Check sheet for the modelled part. Datum: model origin and axes. Units: mm. Face numbers are marked on the shaded views. A direction names the side the tool comes from. Round coordinates to 2 decimals unless told otherwise and drop trailing zeros. Write each loop counter-clockwise with the first axis right and the second up, starting at its lowest first coordinate (ties: lowest second). Pieces come first, ordered by that corner, then holes. Notation, with made-up numbers: (-12, 86) - (43, 86) arc R21 ccw to (43, 108) - close; hole circle Ø2 at (7.25, 23). An arc over 180 degrees is marked (long way). Use one line per item in the form item = value. Start each with the question number.
1) Section check C-C (z = 4.5). Record the boundary of the cut face in (x, y).
2) Section check D-D (x = -17). Record the boundary of the cut face in (y, z), then the cut area to 3 significant figures.
3) Gauge pin test, flat ends, axial feed: P1, Ø3, axis at y = -4.5, z = 8.5, coming from the -X side; P2, Ø1, axis at y = 10, z = 12, coming from the +X side; P3, Ø6, axis at x = -1.5, z = 12.5, coming from the -Y side; P4, Ø15, axis at x = 0, y = 0, coming from the +Z side. Record the tip position at first contact, or that the pin passes through.
4) Section check A-A (x = -6.5). Record the boundary of the cut face in (y, z).
5) Set-up check for the marked faces 1 and 2: record each of +Z, -Z, +X, -X, +Y, -Y from which the full face is reachable in a straight line by a thin tool's end or side.
6) Section check B-B (y = 3.5). Record the boundary of the cut face in (x, z), then the cut area to 3 significant figures.
7) Scan lines: probe 1 along X at (y, z) = (0, 6.5); probe 2 along X at (y, z) = (6.5, 1.75). Record each from-to range of solid material in increasing order.
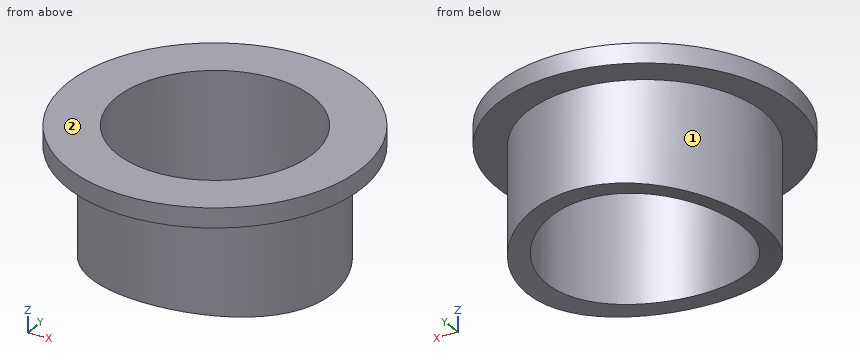
from build123d import *

# Parameters (mm, degrees)
F0_W          = 2.54
F0_H          = 12.7
F3_DEPTH      = 25.4
F2_R          = 69.85
F4_DEPTH      = 25.4
F4_DEPTH_BACK = 25.4


with BuildPart() as f1:
    # F0 (on Front) → F1 (revolve)
    with BuildSketch(Plane.XZ):
        with Locations((-13.97, 6.35)):
            Rectangle(F0_W, F0_H)
        Polygon((-15.24, 12.7), (-12.7, 12.7), (-12.7, 15.24), (-19.05, 15.24), (-19.05, 12.7), align=None)
    revolve(axis=Axis((0, 0, 10.1733254269), (0, 0, 1)))

    # F3 (add): a face of the model
    f3_faces = [f1.faces().sort_by_distance(p)[0] for p in [
        (14.8089477062, 0, 0),
    ]]
    extrude(f3_faces, amount=F3_DEPTH)

    # F2 (on Front) → F4 (cut, two sides)
    with BuildSketch(Plane.XZ) as f4_sk:
        with Locations((0, -69.85)):
            Circle(F2_R)
    extrude(amount=-F4_DEPTH, mode=Mode.SUBTRACT)
    extrude(f4_sk.sketch, amount=F4_DEPTH_BACK, mode=Mode.SUBTRACT)


solid = f1.part
Results are:
q1.outline = circle Ø30.48 at (0, 0); hole circle Ø25.4 at (0, 0)
q2.outline = (-8.6, 12.7) - (8.6, 12.7) - (8.6, 15.24) - (-8.6, 15.24) - close
q2.area = 43.7 mm²
q3.P1 = -14.94
q3.P2 = 11.92
q3.P3 = -19.05
q3.P4 = through
q4.outline = (-17.91, 12.7) - (-13.78, 12.7) - (-13.78, -0.3) - (-10.91, -0.3) - (-10.91, 15.24) - (-17.91, 15.24) - close; (10.91, -0.3) - (13.78, -0.3) - (13.78, 12.7) - (17.91, 12.7) - (17.91, 15.24) - (10.91, 15.24) - close
q5.face_1 = -Z
q5.face_2 = +Z, +X, -X, +Y, -Y
q6.outline = (-18.73, 12.7) - (-14.83, 12.7) - (-14.83, -1.59) arc R69.85 cw to (-12.21, -1.08) - (-12.21, 15.24) - (-18.73, 15.24) - close; (12.21, -1.08) arc R69.85 cw to (14.83, -1.59) - (14.83, 12.7) - (18.73, 12.7) - (18.73, 15.24) - (12.21, 15.24) - close
q6.area = 107 mm²
q7.probe_1 = -15.24 to -12.7, 12.7 to 15.24
q7.probe_2 = -13.78 to -10.91, 10.91 to 13.78
